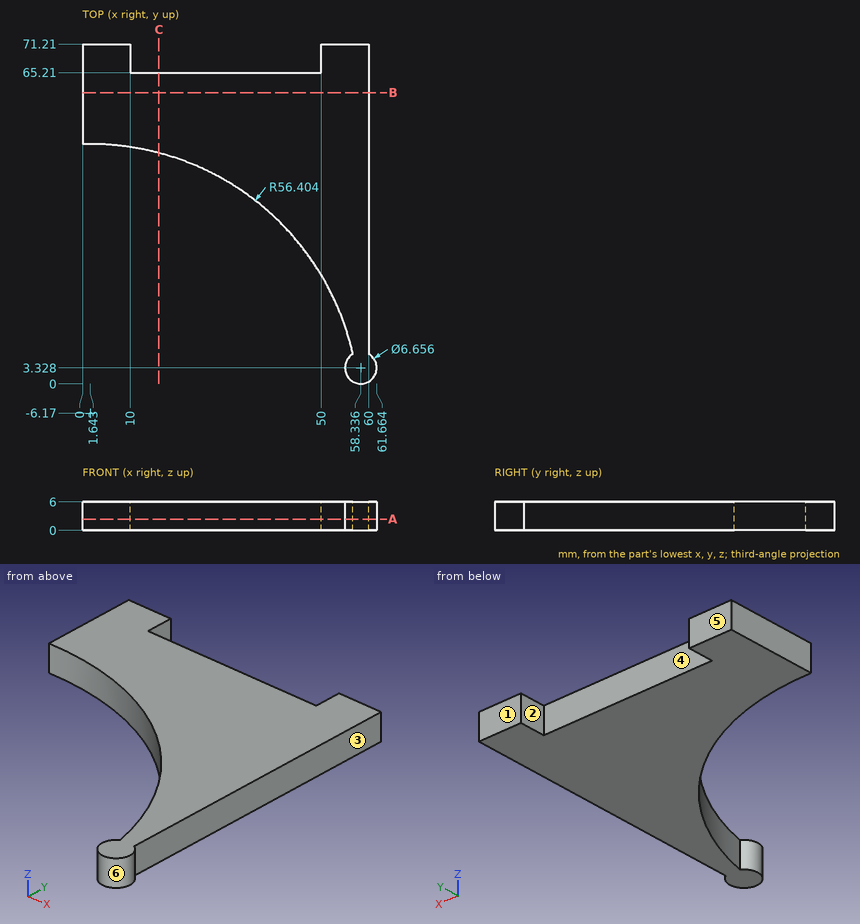
Print and shaded views of the part. All mm, measured from the part's lowest x, y and z. A direction names the side the tool comes from. Coordinates: 2 decimals unless noted, no trailing zeros. Loops run counter-clockwise (first coordinate to the right, second up) from the corner with the lowest first, then second, coordinate; pieces in that order, holes last. Notation, with made-up numbers: (18, 86.5) - (57, 86.5) arc R25 ccw to (57, 112.5) - close; hole circle Ø10 at (22, -39.75). An arc over 180 degrees is marked (long way). Write item = value, one per line. Start each with the question number.
Item 1: Cut at A-A, the plane z = 2.35. Give the cut face in (x, y) (1 decimal), and give its area (3 significant figures).
Item 2: Cut at B-B, the plane y = 61. Give the cut face in (x, z), and give its area (3 significant figures).
Item 3: Wall check: L1, parallel to X at y = 55, z = 1.7; L2, parallel to X at y = 66, z = 4.55; L3, parallel to X at y = 8.5, z = 0.55 (1 decimal). Give the ranges that are in metal, low to high. Write a range as from..to.
Item 4: Cut at C-C, the plane x = 16. Give the cut face in (y, z).
Item 5: 3-axis set-ups, long thin cutter, end or side, ignore diameter. For the marked faces 1, 2 and 3: which of +Z, -Z, +X, -X, +Y, -Y reach the whole face in a straight line?
Item 6: Mould opens along X. For the marked faces 4, 5 and 6 say: released by +X, released by -X, zero draft, split by the parting line, or undercut.
Item 7: Flat gauge pins, fed straight in: pin 1 Ø1.5 at (y, z) = (16, 1.5) entering from +X; pin 2 Ø1 at (x, z) = (45.5, 4) entering from -Y; pin 3 Ø3 at (x, z) = (21, 4) entering from +Y. Where does each tip first touch, or does it go through?
The answers:
q1.outline = (0, 50.2) arc R56.4 cw to (56.7, 6.2) arc R3.3 ccw (long way) to (60, 6.2) - (60, 71.2) - (50, 71.2) - (50, 65.2) - (10, 65.2) - (10, 71.2) - (0, 71.2) - close
q1.area = 1,820 mm2
q2.outline = (0, 0) - (60, 0) - (60, 6) - (0, 6) - close
q2.area = 360 mm2
q3.L1 = 0..60
q3.L2 = 0..10, 50..60
q3.L3 = 56.1..60
q4.outline = (48.38, 0) - (65.21, 0) - (65.21, 6) - (48.38, 6) - close
q5.face_1 = +Z, -Z, +X, -X, +Y
q5.face_2 = +Z, -Z, +Y
q5.face_3 = +Z, -Z, +X, +Y
q6.face_4 = undercut
q6.face_5 = zero draft
q6.face_6 = split by the parting line
q7.pin_1 = 60
q7.pin_2 = 28.67
q7.pin_3 = 65.21
